Source: CAD feature listing. Evaluate the final solid. Frame: model axes, mm. A direction names the side the tool comes from. Give positions to 0.01 mm unless a question says otherwise; leave off trailing zeros. Order: outer loops, then holes, each group sorted by start corner. A loop starts at its lowest first (then second) coordinate and runs counter-clockwise, first axis right, second up. Notation, with made-up numbers: M 41,76.5 L 56,76.5 A18 cw 56,99.5 Z; hole C -30,-38 d10. An arc over 180 degrees is marked long. Return JSON: item names as keys, results as strings.
from build123d import *

# Parameters (mm, degrees)
SKETCH1_R           = 10
SKETCH1_R_2         = 3.1
SKETCH1_R_3         = 1.45
BOSS_EXTRUDE1_DEPTH = 7
SKETCH8_R           = 5.25
SKETCH8_R_2         = 3.1
BOSS_EXTRUDE4_DEPTH = 1
CUT_EXTRUDE1_DEPTH  = 3.2
CUT_EXTRUDE2_DEPTH  = 4.2


with BuildPart() as part:
    # Sketch1 → Boss-Extrude1 (new body)
    with BuildSketch(Plane(origin=(0, 0, 0), x_dir=(1, 0, 0), z_dir=(0, 1, 0))):
        Circle(SKETCH1_R)
        Circle(SKETCH1_R_2, mode=Mode.SUBTRACT)
        with Locations((0, 7)):
            Circle(SKETCH1_R_3, mode=Mode.SUBTRACT)
        with Locations((7, 0)):
            Circle(SKETCH1_R_3, mode=Mode.SUBTRACT)
        with Locations((0, -7)):
            Circle(SKETCH1_R_3, mode=Mode.SUBTRACT)
        with Locations((-7, 0)):
            Circle(SKETCH1_R_3, mode=Mode.SUBTRACT)
    extrude(amount=BOSS_EXTRUDE1_DEPTH)

    # Sketch8 → Boss-Extrude4 (add)
    with BuildSketch(Plane.XZ):
        Circle(SKETCH8_R)
        Circle(SKETCH8_R_2, mode=Mode.SUBTRACT)
    extrude(amount=BOSS_EXTRUDE4_DEPTH)

    # Sketch9 → Cut-Extrude1 (cut)
    with BuildSketch(Plane.XZ.offset(1)):
        with BuildLine():
            Line((-7, 2.85), (-9.585275166, 2.85))
            ThreePointArc((-9.585275166, 2.85), (-10, 0), (-9.585275166, -2.85))
            Line((-9.585275166, -2.85), (-7, -2.85))
            ThreePointArc((-7, -2.85), (-5.845254282, -2.605582915), (-4.888571429, -1.914254264))
            ThreePointArc((-4.888571429, -1.914254264), (-5.25, 0), (-4.888571429, 1.914254264))
            ThreePointArc((-4.888571429, 1.914254264), (-5.845254282, 2.605582915), (-7, 2.85))
        make_face()
        with BuildLine():
            Line((-2.85, 9.585275166), (-2.85, 7))
            ThreePointArc((-2.85, 7), (-2.605582915, 5.845254282), (-1.914254264, 4.888571429))
            ThreePointArc((-1.914254264, 4.888571429), (0, 5.25), (1.914254264, 4.888571429))
            ThreePointArc((1.914254264, 4.888571429), (2.605582915, 5.845254282), (2.85, 7))
            Line((2.85, 7), (2.85, 9.585275166))
            ThreePointArc((2.85, 9.585275166), (0, 10), (-2.85, 9.585275166))
        make_face()
        with BuildLine():
            ThreePointArc((10, 0), (9.895775656, 1.440008393), (9.585275166, 2.85))
            Line((9.585275166, 2.85), (7, 2.85))
            ThreePointArc((7, 2.85), (5.845254282, 2.605582915), (4.888571429, 1.914254264))
            ThreePointArc((4.888571429, 1.914254264), (5.158851616, 0.974037987), (5.25, 0))
            ThreePointArc((5.25, 0), (5.158851616, -0.974037987), (4.888571429, -1.914254264))
            ThreePointArc((4.888571429, -1.914254264), (5.845254282, -2.605582915), (7, -2.85))
            Line((7, -2.85), (9.585275166, -2.85))
            ThreePointArc((9.585275166, -2.85), (9.895775656, -1.440008393), (10, 0))
        make_face()
        with BuildLine():
            Line((-2.85, -7), (-2.85, -9.585275166))
            ThreePointArc((-2.85, -9.585275166), (0, -10), (2.85, -9.585275166))
            Line((2.85, -9.585275166), (2.85, -7))
            ThreePointArc((2.85, -7), (2.605582915, -5.845254282), (1.914254264, -4.888571429))
            ThreePointArc((1.914254264, -4.888571429), (0, -5.25), (-1.914254264, -4.888571429))
            ThreePointArc((-1.914254264, -4.888571429), (-2.605582915, -5.845254282), (-2.85, -7))
        make_face()
        with BuildLine():
            ThreePointArc((-4.888571429, -1.914254264), (-4.15, 0), (-4.888571429, 1.914254264))
            ThreePointArc((-4.888571429, 1.914254264), (-5.25, 0), (-4.888571429, -1.914254264))
        make_face()
        with BuildLine():
            ThreePointArc((1.914254264, 4.888571429), (0, 5.25), (-1.914254264, 4.888571429))
            ThreePointArc((-1.914254264, 4.888571429), (0, 4.15), (1.914254264, 4.888571429))
        make_face()
        with BuildLine():
            ThreePointArc((5.25, 0), (5.158851616, 0.974037987), (4.888571429, 1.914254264))
            ThreePointArc((4.888571429, 1.914254264), (4.15, 0), (4.888571429, -1.914254264))
            ThreePointArc((4.888571429, -1.914254264), (5.158851616, -0.974037987), (5.25, 0))
        make_face()
        with BuildLine():
            ThreePointArc((1.914254264, -4.888571429), (0, -4.15), (-1.914254264, -4.888571429))
            ThreePointArc((-1.914254264, -4.888571429), (0, -5.25), (1.914254264, -4.888571429))
        make_face()
    extrude(amount=-CUT_EXTRUDE1_DEPTH, mode=Mode.SUBTRACT)

    # Sketch10 → Cut-Extrude2 (cut)
    with BuildSketch(Plane(origin=(0, 7, 0), x_dir=(1, 0, 0), z_dir=(0, 1, 0))):
        Polygon((1.464406605, 5.465239851), (-4.000833247, 4.000833247), (-5.465239851, -1.464406605), (-1.464406605, -5.465239851), (4.000833247, -4.000833247), (5.465239851, 1.464406605), align=None)
    extrude(amount=-CUT_EXTRUDE2_DEPTH, mode=Mode.SUBTRACT)


solid = part.part
1. Section query D-D (y = 1.25). Return loops of the section in (x, z).
Evaluation:
{"outline": "M -9.59,-2.85 A10 ccw -2.85,-9.59 L -2.85,-7 A2.85 cw 2.85,-7 L 2.85,-9.59 A10 ccw 9.59,-2.85 L 7,-2.85 A2.85 cw 7,2.85 L 9.59,2.85 A10 ccw 2.85,9.59 L 2.85,7 A2.85 cw -2.85,7 L -2.85,9.59 A10 ccw -9.59,2.85 L -7,2.85 A2.85 cw -7,-2.85 Z; hole C 0,0 d6.2"}
2. Draft query along X for faces 1 (the face through (3.691, -0.493, -3.734)), 2 (the face through (1.2, 2.2, -8.3)), 3 (the face through (-8, 1, -2.85)), 4 (the face through (1.23, 4.929, 4.743)). Return one class per face: pulls with the +X half, pulls with the -X half, needs draft (parallel to the pull), parting line crosses it, or undercut.
Evaluation:
{"face 1": "pulls with the +X half", "face 2": "undercut", "face 3": "needs draft", "face 4": "undercut"}
3. Ray query, probe 1 along X at (y, z) = (3.5, 0); probe 2 along Y at (x, z) = (-3.75, -3.5); probe 3 along Y at (x, z) = (8.5, 4.5). Return the intervals inside material, ascending.
Evaluation:
{"probe 1": "x = -10 to -8.45, -5.55 to -5.07, 5.07 to 5.55, 8.45 to 10", "probe 2": "y = -1 to 2.8", "probe 3": "y = 0 to 7"}
4. Set-up query: faces 5 (the face through (-1.23, 4.929, -4.743)), 6 (the face through (8, 1, -2.85)), 7 (the face through (-2.85, 1, -8)), 8 (the face through (-2.85, 1, 8)). Return all of +Z, -Z, +X, -X, +Y, -Y with unobstructed straight access to the full face (end or side cutting, diameter ignored); none if empty.
Evaluation:
{"face 5": "+Y", "face 6": "+X, -Y", "face 7": "-Z, -Y", "face 8": "+Z, -Y"}
5. First-contact query: pin 1 (1.5 mm diameter, centred on x = -7, z = 4, fed in from -Y); pin 2 (1.1 mm diameter, centred on y = 1, z = -8, fed in from -X); pin 3 (0.7 mm diameter, centred on y = 1.5, z = -8.5, fed in from +X). Flat tips, straight axial feed; report the tip coordinate or a pass-through.
Evaluation:
{"pin 1": "stops at y = 0", "pin 2": "stops at x = -6.67", "pin 3": "stops at x = 5.79"}
6. Section query C-C (x = 0). Return loops of the section in (y, z), then the cut area to 3 significant figures.
Evaluation:
{"outline": "M -1,-4.15 L 2.2,-4.15 L 2.2,-5.55 L 7,-5.55 L 7,-5.07 L 2.8,-5.07 L 2.8,-3.1 L -1,-3.1 Z; M -1,3.1 L 2.8,3.1 L 2.8,5.07 L 7,5.07 L 7,5.55 L 2.2,5.55 L 2.2,4.15 L -1,4.15 Z; M 2.2,-10 L 7,-10 L 7,-8.45 L 2.2,-8.45 Z; M 2.2,8.45 L 7,8.45 L 7,10 L 2.2,10 Z", "area": "28.5 mm^2"}
7. Section query A-A (y = 5). Return loops of the section in (x, z), then the cut area to 3 significant figures.
Evaluation:
{"outline": "C 0,0 d20; hole C -7,0 d2.9; hole M -5.47,1.46 L -4,-4 L 1.46,-5.47 L 5.47,-1.46 L 4,4 L -1.46,5.47 Z; hole C 0,-7 d2.9; hole C 0,7 d2.9; hole C 7,0 d2.9", "area": "205 mm^2"}
8. Section query B-B (z = 0.5). Return loops of the section in (x, y).
Evaluation:
{"outline": "M -9.99,2.2 L -8.36,2.2 L -8.36,7 L -9.99,7 Z; M -5.64,2.2 L -4.19,2.2 L -4.19,-1 L -3.06,-1 L -3.06,2.8 L -5.21,2.8 L -5.21,7 L -5.64,7 Z; M 3.06,-1 L 4.19,-1 L 4.19,2.2 L 5.64,2.2 L 5.64,7 L 4.94,7 L 4.94,2.8 L 3.06,2.8 Z; M 8.36,2.2 L 9.99,2.2 L 9.99,7 L 8.36,7 Z"}
